Geometry check sheet. Reference: drawing and pictorial views, mm from the part's lowest x, y, z. A direction names the side the tool comes from. Coordinates: 2 decimals unless noted, no trailing zeros. Loops run counter-clockwise (first coordinate to the right, second up) from the corner with the lowest first, then second, coordinate; pieces in that order, holes last. Notation, with made-up numbers: (-23.5, -25) -> (16.5, -25) arc R32 ccw to (16.5, 12) -> close; hole circle Ø10 at (37, 15.5). An arc over 180 degrees is marked (long way). Use one line per item in the form item = value.
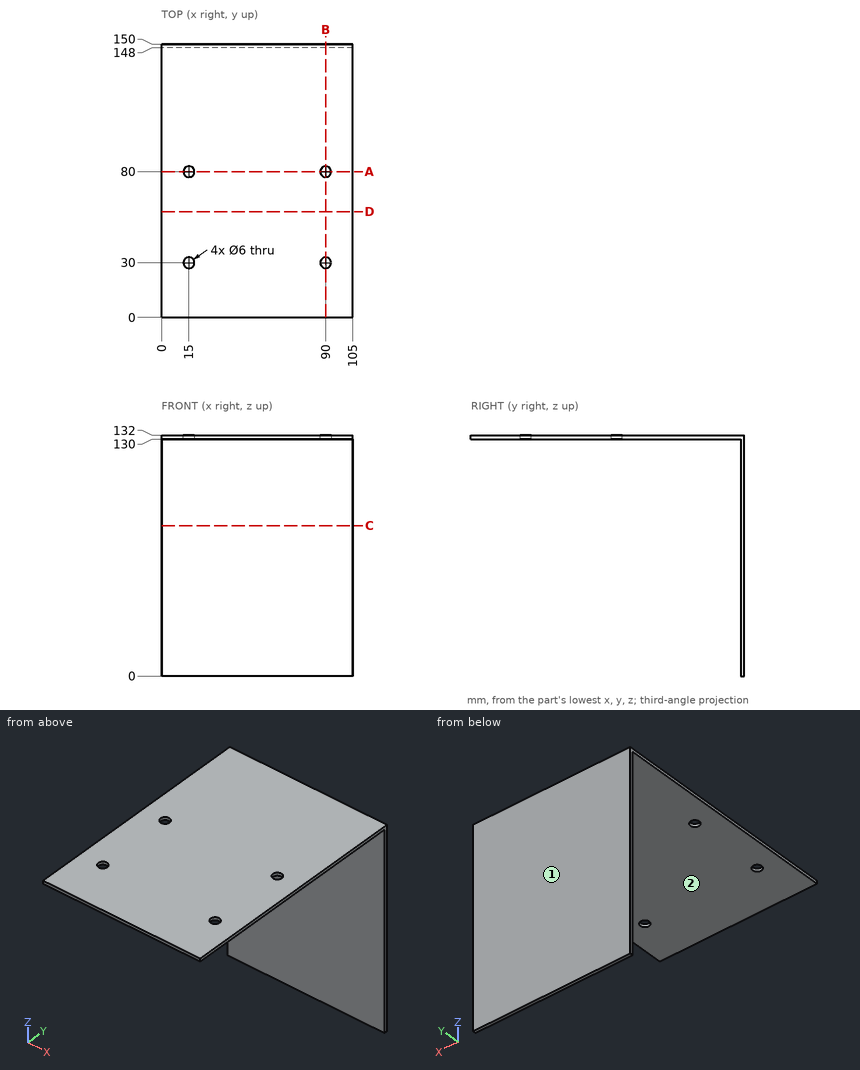
(1) Scan lines: line 1 along Y through (x, z) = (90, 130.5); line 2 along Y through (x, z) = (91, 15.5); line 3 along Z through (x, y) = (15, 72.5). Record each from-to range of solid material in increasing order.
Established:
line_1 = 0 to 27, 33 to 77, 83 to 150
line_2 = 148 to 150
line_3 = 130 to 132
(2) Tool access check on the marked faces 1 and 2. Record the directions out of +Z, -Z, +X, -X, +Y, -Y that give a thin tool (end or side, any length) a straight path to the whole face; none if there is none.
Established:
face_1 = +Z, -Z, +X, -X, +Y
face_2 = -Z, +X, -X, -Y
(3) Section check D-D, the plane y = 58. Record the boundary of the cut face in (x, z).
Established:
outline = (0, 130) -> (105, 130) -> (105, 132) -> (0, 132) -> close
(4) Section check B-B, the plane x = 90. Record the boundary of the cut face in (y, z).
Established:
outline = (0, 130) -> (27, 130) -> (27, 132) -> (0, 132) -> close; (33, 130) -> (77, 130) -> (77, 132) -> (33, 132) -> close; (83, 130) -> (148, 130) -> (148, 0) -> (150, 0) -> (150, 132) -> (83, 132) -> close
(5) Go/stop test with flat-tipped pins: P1, Ø3.5, axis at x = 15, y = 80, coming from the -Z side; P2, Ø5, axis at x = 24, y = 101.5, coming from the -Z side; P3, Ø10, axis at x = 81, z = 36, coming from the -Y side. Record where each tip stops, or that it passes through.
Established:
P1 = through
P2 = 130
P3 = 148
(6) Section check A-A, the plane y = 80. Record the boundary of the cut face in (x, z), plus the area to 3 significant figures.
Established:
outline = (0, 130) -> (12, 130) -> (12, 132) -> (0, 132) -> close; (18, 130) -> (87, 130) -> (87, 132) -> (18, 132) -> close; (93, 130) -> (105, 130) -> (105, 132) -> (93, 132) -> close
area = 186 mm²
(7) Section check C-C, the plane z = 82.5. Record the boundary of the cut face in (x, y), plus the area to 3 significant figures.
Established:
outline = (0, 148) -> (105, 148) -> (105, 150) -> (0, 150) -> close
area = 210 mm²
